Geometry: final body of the model. Coordinates: model frame, mm. Face numbers are marked on the shaded views. A direction names the side the tool comes from. Coordinates: 2 decimals unless noted, no trailing zeros. Loops run counter-clockwise (first coordinate to the right, second up) from the corner with the lowest first, then second, coordinate; pieces in that order, holes last. Notation, with made-up numbers: (-14.5, 89.25) - (14.5, 89.25) arc R11 ccw to (14.5, 108.25) - close; hole circle Ø4 at (8, 29). An arc over 180 degrees is marked (long way). Answer in a Markdown table with one row per item.
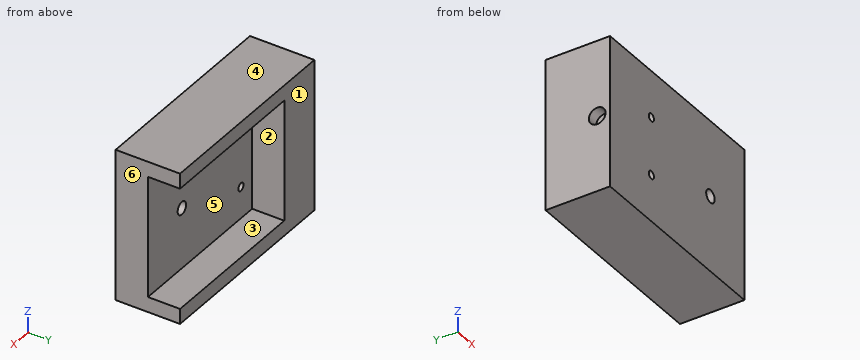
from build123d import *

# Parameters (mm, degrees)
SKETCH1_W           = 91
SKETCH1_H           = 67.9
BOSS_EXTRUDE1_DEPTH = 28.9
SKETCH2_W           = 70.6
SKETCH2_H           = 54.3
CUT_EXTRUDE1_DEPTH  = 14.4
SKETCH3_R           = 3.75
CUT_EXTRUDE2_DEPTH  = 5
SKETCH4_R           = 2.871512345
SKETCH4_R_2         = 1.754658852
CUT_EXTRUDE3_DEPTH  = 14.5


with BuildPart() as part:
    # Sketch1 → Boss-Extrude1 (new body)
    with BuildSketch(Plane(origin=(0, 0, 0), x_dir=(1, 0, 0), z_dir=(0, 1, 0))):
        Rectangle(SKETCH1_W, SKETCH1_H)
    extrude(amount=BOSS_EXTRUDE1_DEPTH)

    # Sketch2 → Cut-Extrude1 (cut)
    with BuildSketch(Plane(origin=(0, 28.9, 0), x_dir=(1, 0, 0), z_dir=(0, 1, 0))):
        with Locations((10.2, 0)):
            Rectangle(SKETCH2_W, SKETCH2_H)
    extrude(amount=-CUT_EXTRUDE1_DEPTH, mode=Mode.SUBTRACT)

    # Sketch3 → Cut-Extrude2 (cut)
    with BuildSketch(Plane.ZY.offset(45.5)):
        with Locations((0, 5.750396788)):
            Circle(SKETCH3_R)
    extrude(amount=-CUT_EXTRUDE2_DEPTH, mode=Mode.SUBTRACT)

    # Sketch4 → Cut-Extrude3 (cut)
    with BuildSketch(Plane(origin=(0, 14.5, 0), x_dir=(1, 0, 0), z_dir=(0, 1, 0))):
        with Locations(Location((22.5, 0, 0), (0, 0, 270))):
            Circle(SKETCH4_R)
        with Locations(Location((-17.5, 13, 0), (0, 0, 270))):
            Circle(SKETCH4_R_2)
        with Locations(Location((-17.5, -13, 0), (0, 0, 270))):
            Circle(SKETCH4_R_2)
    extrude(amount=-CUT_EXTRUDE3_DEPTH, mode=Mode.SUBTRACT)


solid = part.part
(1) First-contact query: pin 1 Ø3.5 at (x, z) = (22.5, 0) entering from -Y; pin 2 Ø6 at (x, z) = (35.5, -24.5) entering from +Y; pin 3 Ø7 at (y, z) = (24, 12.5) entering from +X; pin 4 Ø10 at (x, z) = (-3.5, 21) entering from +Y. Flat tips, straight axial feed; report the tip coordinate or a pass-through.
Verdict:
| item | result |
|---|---|
| pin 1 | passes through |
| pin 2 | stops at y = 28.9 |
| pin 3 | stops at x = -25.1 |
| pin 4 | stops at y = 14.5 |
(2) Cut plane D-D on x = 32.5. Output: boundary loops of the cut face in (y, z).
Verdict:
| item | result |
|---|---|
| outline | (0, -33.95) - (28.9, -33.95) - (28.9, -27.15) - (14.5, -27.15) - (14.5, 27.15) - (28.9, 27.15) - (28.9, 33.95) - (0, 33.95) - close |
(3) Cut plane B-B on z = 13. Output: boundary loops of the cut face in (x, y), then the cut area to 3 significant figures.
Verdict:
| item | result |
|---|---|
| outline | (-45.5, 0) - (-19.25, 0) - (-19.25, 14.5) - (-25.1, 14.5) - (-25.1, 28.9) - (-45.5, 28.9) - close; (-15.75, 0) - (45.5, 0) - (45.5, 14.5) - (-15.75, 14.5) - close |
| area | 1,560 mm² |
(4) Pull-direction query (Z, two-part tool) for the marked faces 3, 4, 5 and 6; classes: pulls with the +Z half, pulls with the -Z half, needs draft (parallel to the pull), parting line crosses it, or undercut.
Verdict:
| item | result |
|---|---|
| face 3 | undercut |
| face 4 | pulls with the +Z half |
| face 5 | undercut |
| face 6 | needs draft |
(5) Ray query, probe 1 along X at (y, z) = (4, 13); probe 2 along Z at (x, y) = (9.5, 21.5); probe 3 along X at (y, z) = (5, 0). Return the intervals inside material, ascending.
Verdict:
| item | result |
|---|---|
| probe 1 | x = -45.5 to -19.25, -15.75 to 45.5 |
| probe 2 | z = -33.95 to -27.15, 27.15 to 33.95 |
| probe 3 | x = -40.5 to 19.63, 25.37 to 45.5 |
(6) Access query for the marked faces 1 and 2. Directions: +Z, -Z, +X, -X, +Y, -Y. A direction counts if a zero-diameter tool reaches every point of the face in a straight line with its end or side. Return the directions, or none.
Verdict:
| item | result |
|---|---|
| face 1 | +Z, -Z, +X, -X, +Y |
| face 2 | +X, +Y |
(7) Cut plane C-C on x = -17.5. Output: boundary loops of the cut face in (y, z), then the cut area to 3 significant figures.
Verdict:
| item | result |
|---|---|
| outline | (0, -33.95) - (28.9, -33.95) - (28.9, -27.15) - (14.5, -27.15) - (14.5, -14.75) - (0, -14.75) - close; (0, -11.25) - (14.5, -11.25) - (14.5, 11.25) - (0, 11.25) - close; (0, 14.75) - (14.5, 14.75) - (14.5, 27.15) - (28.9, 27.15) - (28.9, 33.95) - (0, 33.95) - close |
| area | 1,080 mm² |
(8) Cut plane A-A on x = 22.5. Output: boundary loops of the cut face in (y, z), then the cut area to 3 significant figures.
Verdict:
| item | result |
|---|---|
| outline | (0, -33.95) - (28.9, -33.95) - (28.9, -27.15) - (14.5, -27.15) - (14.5, -2.87) - (0, -2.87) - close; (0, 2.87) - (14.5, 2.87) - (14.5, 27.15) - (28.9, 27.15) - (28.9, 33.95) - (0, 33.95) - close |
| area | 1,100 mm² |
